```python
from build123d import *

# Parameters (mm, degrees)
EXTRUDE_1_DEPTH        = 2
EXTRUDE_2_DEPTH        = 2
CUT_EXTRUDE_1_REACH    = 40.942
PATTERN_LINEAR_1_COUNT = 2
PATTERN_LINEAR_1_PITCH = 15
CUT_EXTRUDE_2_REACH    = 40.942
FILLET_1_R             = 0.2


with BuildPart() as part:
    # 草图1 → 凸台-拉伸1 (new body)
    with BuildSketch(Plane(origin=(0, 0, 0), x_dir=(1, 0, 0), z_dir=(0, 1, 0))):
        Polygon((0, 0), (0, -27.5), (10, -27.5), (10, -10), (27.5, -10), (27.5, 0), align=None)
    extrude(amount=EXTRUDE_1_DEPTH)

    # 草图2 → 凸台-拉伸2 (add)
    with BuildSketch(Plane(origin=(0, 2, 0), x_dir=(1, 0, 0), z_dir=(0, 1, 0))):
        with BuildLine():
            Line((27, 0), (16, 0))
            ThreePointArc((16, 0), (15.5, -0.5), (16, -1))
            Line((16, -1), (27, -1))
            ThreePointArc((27, -1), (27.5, -0.5), (27, 0))
        make_face()
        with BuildLine():
            Line((27, -9), (16, -9))
            ThreePointArc((16, -9), (15.5, -9.5), (16, -10))
            Line((16, -10), (27, -10))
            ThreePointArc((27, -10), (27.5, -9.5), (27, -9))
        make_face()
        with BuildLine():
            Line((1, -27), (1, -16))
            ThreePointArc((1, -16), (0.5, -15.5), (0, -16))
            Line((0, -16), (0, -27))
            ThreePointArc((0, -27), (0.5, -27.5), (1, -27))
        make_face()
        with BuildLine():
            Line((9, -27), (9, -16))
            ThreePointArc((9, -16), (9.5, -15.5), (10, -16))
            Line((10, -16), (10, -27))
            ThreePointArc((10, -27), (9.5, -27.5), (9, -27))
        make_face()
    extrude(amount=EXTRUDE_2_DEPTH)

    # 草图3 → 切除-拉伸1 (cut, up to next)
    with BuildSketch(Plane(origin=(0, 2, 0), x_dir=(1, 0, 0), z_dir=(0, 1, 0)), mode=Mode.PRIVATE) as cut_extrude_1_sk1:
        with BuildLine():
            Line((23.5, -3.5), (23.5, -6.5))
            Line((23.5, -6.5), (21.322875656, -6.5))
            ThreePointArc((21.322875656, -6.5), (20, -7), (18.677124344, -6.5))
            Line((18.677124344, -6.5), (16.5, -6.5))
            Line((16.5, -6.5), (16.5, -3.5))
            Line((16.5, -3.5), (18.677124344, -3.5))
            ThreePointArc((18.677124344, -3.5), (20, -3), (21.322875656, -3.5))
            Line((21.322875656, -3.5), (23.5, -3.5))
        make_face()
    cut_extrude_1_tool1 = extrude(cut_extrude_1_sk1.sketch, amount=-CUT_EXTRUDE_1_REACH, mode=Mode.PRIVATE) & part.part
    cut_extrude_1 = cut_extrude_1_tool1.solids().sort_by_distance((20, 2, 5))[0]
    add(cut_extrude_1, mode=Mode.SUBTRACT)

    # 阵列(线性)1: 切除-拉伸1 ×2
    with Locations(*[(-i * PATTERN_LINEAR_1_PITCH, 0, 0) for i in range(1, PATTERN_LINEAR_1_COUNT)]):
        add(cut_extrude_1, mode=Mode.SUBTRACT)

    # 草图4 → 切除-拉伸2 (cut, up to next)
    with BuildSketch(Plane(origin=(0, 2, 0), x_dir=(1, 0, 0), z_dir=(0, 1, 0)), mode=Mode.PRIVATE) as cut_extrude_2_sk1:
        with BuildLine():
            Line((6.5, -23.5), (3.5, -23.5))
            Line((3.5, -23.5), (3.5, -21.322875656))
            ThreePointArc((3.5, -21.322875656), (3, -20), (3.5, -18.677124344))
            Line((3.5, -18.677124344), (3.5, -16.5))
            Line((3.5, -16.5), (6.5, -16.5))
            Line((6.5, -16.5), (6.5, -18.677124344))
            ThreePointArc((6.5, -18.677124344), (7, -20), (6.5, -21.322875656))
            Line((6.5, -21.322875656), (6.5, -23.5))
        make_face()
    cut_extrude_2_tool1 = extrude(cut_extrude_2_sk1.sketch, amount=-CUT_EXTRUDE_2_REACH, mode=Mode.PRIVATE) & part.part
    add(cut_extrude_2_tool1.solids().sort_by_distance((5, 2, 20))[0], mode=Mode.SUBTRACT)

    # 圆角1
    fillet_1_edges = [part.edges().sort_by_distance(p)[0] for p in [
        (27.5, 1, 0),
        (27.5, 1, 10),
        (0, 1, 27.5),
        (10, 1, 27.5),
        (5, 0, 27.5),
        (27.5, 0, 5),
        (10, 0, 18.75),
        (18.75, 0, 10),
        (0, 0, 13.75),
        (13.75, 0, 0),
    ]]
    fillet(fillet_1_edges, radius=FILLET_1_R)


solid = part.part
```
Here's how the part is built. I have some questions about the finished solid (model axes, mm). A direction names the side the tool comes from. Round coordinates to 2 decimals unless told otherwise and drop trailing zeros. Order: outer loops, then holes, each group sorted by start corner. A loop starts at its lowest first (then second) coordinate and runs counter-clockwise, first axis right, second up. Notation, with made-up numbers: M -39,71.25 L -17,71.25 A18 ccw -17,98.25 Z; hole C 80,-9 d8. An arc over 180 degrees is marked long. Answer in a Markdown table with one row per item.
Item 1: Imagine slicing it at C-C, the plane x = 5. Write out the boundary of the cut face in (y, z), and give its area (3 significant figures).
A:
| item | result |
|---|---|
| outline | M 0,0.2 A0.2 ccw 0.2,0 L 2,0 L 2,3 L 0,3 Z; M 0,7 L 2,7 L 2,16.5 L 0,16.5 Z; M 0,23.5 L 2,23.5 L 2,27.5 L 0.2,27.5 A0.2 ccw 0,27.3 Z |
| area | 33.0 mm2 |
Item 2: Imagine slicing it at A-A, the plane z = 4.5. Write out the boundary of the cut face in (x, y).
A:
| item | result |
|---|---|
| outline | M 0,0.2 A0.2 ccw 0.2,0 L 1.5,0 L 1.5,2 L 0,2 Z; M 8.5,0 L 16.5,0 L 16.5,2 L 8.5,2 Z; M 23.5,0 L 27.3,0 A0.2 ccw 27.5,0.2 L 27.5,2 L 23.5,2 Z |
Item 3: For faces 4 (the face through (15.5, 3, 0.5)), 5 (the face through (27.5, 3, 9.5)), 6 (the face through (3.5, 1, 18)), 7 (the face through (0.5, 3, 27.5)), 8 (the face through (1, 3, 22)), which set-ups out of +Z, -Z, +X, -X, +Y, -Y let a thin tool reach every point of the face, with its end or its side?
A:
| item | result |
|---|---|
| face 4 | -X, +Y |
| face 5 | +X, +Y |
| face 6 | +Y, -Y |
| face 7 | +Z, +Y |
| face 8 | +Z, -Z, +Y |
Item 4: Imagine slicing it at B-B, the plane y = 0.8. State how many separate pieces and enclosed holes the cut face has, and give its area (3 significant figures).
A:
| item | result |
|---|---|
| separate pieces | 1 |
| enclosed holes | 3 |
| area | 382 mm2 |
Item 5: Thinking about a two-plate mould opening in Z: for faces 1 (the face through (10, 2, 21)), 2 (the face through (17, 2, 0)), 3 (the face through (6.5, 1, 22)), which applies, +Z half, -Z half, draft (parallel to the pull), parting line (faces both ways), or undercut?
A:
| item | result |
|---|---|
| face 1 | draft |
| face 2 | -Z half |
| face 3 | undercut |
Item 6: If I drill on L1, parallel to Z at x = 21.75, y = 1.1; L2, parallel to X at y = 2.1, z = 21.5, over which ranges is the centre line in solid material (lowest first)? Write a range as from..to.
A:
| item | result |
|---|---|
| L1 | z = 0..3.5, 6.5..10 |
| L2 | x = 0..1, 9..10 |
Item 7: Imagine slicing it at D-D, the plane x = 22.25. Write out the boundary of the cut face in (y, z), and give its area (3 significant figures).
A:
| item | result |
|---|---|
| outline | M 0,0.2 A0.2 ccw 0.2,0 L 4,0 L 4,1 L 2,1 L 2,3.5 L 0,3.5 Z; M 0,6.5 L 2,6.5 L 2,9 L 4,9 L 4,10 L 0.2,10 A0.2 ccw 0,9.8 Z |
| area | 18.0 mm2 |
Item 8: I'm going to push flat-ended pins straight in: pin 1 (1 mm diameter, centred on x = 19, y = 2.5, fed in from +Z); pin 2 (2 mm diameter, centred on y = 2.5, z = 11.5, fed in from +X). Where does each tip first touch, or does it pass through?
A:
| item | result |
|---|---|
| pin 1 | stops at z = 10 |
| pin 2 | stops at x = 10 |
